Study the drawing (mm; zero at the part's minimum x, y, z) and answer. A direction names the side the tool comes from. Give positions to 0.01 mm unless a question says otherwise; leave off trailing zeros. Write each loop counter-clockwise with the first axis right and the second up, starting at its lowest first coordinate (ties: lowest second). Pieces come first, ordered by that corner, then holes. Notation, with made-up numbers: M -17,-40 L 28,-40 A15 ccw 28,-14 Z; hole C 73,-0.5 d11. An arc over 180 degrees is marked long. Use a Markdown table: item, result. Add a question column.
Item 1: A cutting plane is placed at C-C on z = 18.5. Determine the outline of the cut face in (x, y), then the cut area to 3 significant figures.
Item 2: A cutting plane is placed at B-B on x = 32. Determine the outline of the cut face in (y, z), then the cut area to 3 significant figures.
Item 3: Given P1, Ø14, axis at x = 33.5, y = 7.5, coming from the +Z side; P2, Ø12, axis at x = 24, y = 6.5, coming from the +Z side, each flat-ended and moving along its own axis, determine where each tip first touches the part or whether it passes through.
Item 4: Consider probe 1 along Z at (x, y) = (32, 20.25); probe 2 along X at (y, z) = (20.5, 21) (1 decimal); probe 3 along X at (y, z) = (3.75, 23) (1 decimal). Determine where each line is inside the solid, lowest interval first. Write a range as [from, to].
Item 5: For the marked faces 4 and 5, determine the directions among +Z, -Z, +X, -X, +Y, -Y from which every point of the face is accessible in a straight line to the end or side of a thin tool.
Item 6: A cutting plane is placed at A-A on y = 6. Determine the outline of the cut face in (x, z).
Item 7: The mould has two halves that part along Y. Classify the marked faces 1, 2 and 3: pulls with the +Y half, pulls with the -Y half, needs draft (parallel to the pull), parting line crosses it, or undercut.
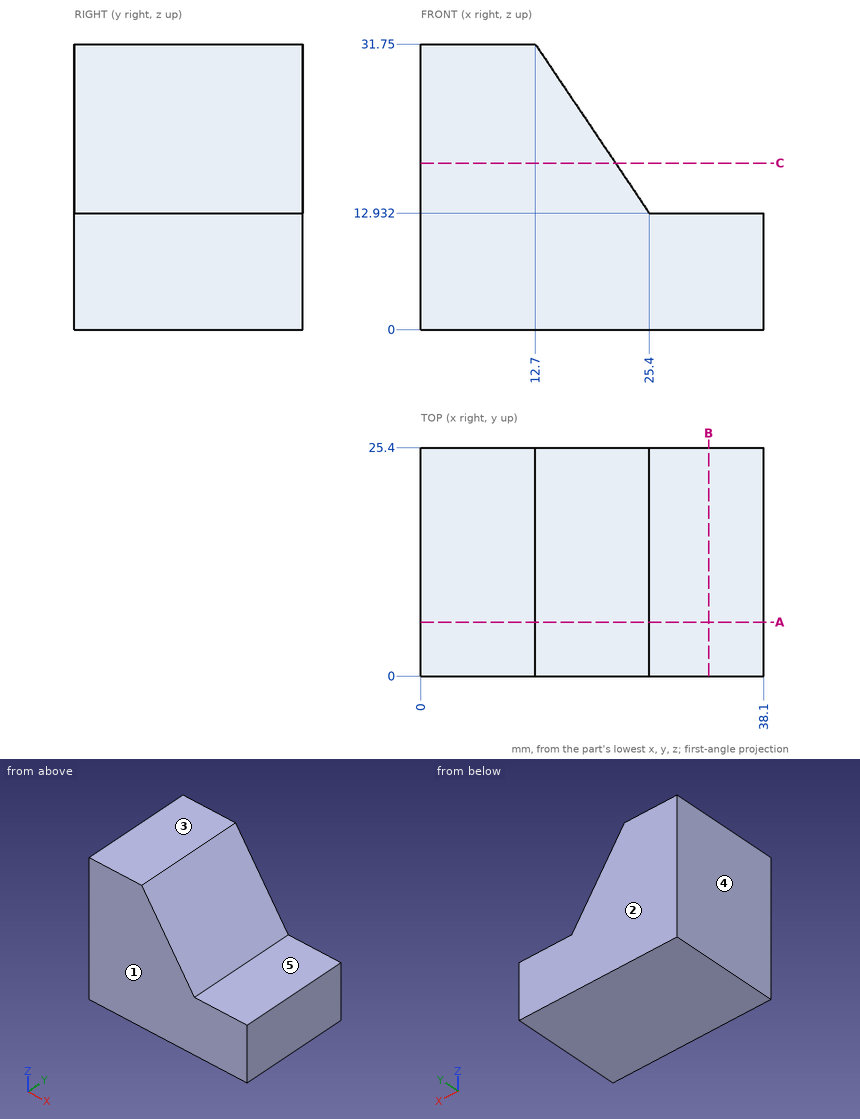
Filled in:
| question | item | result |
|---|---|---|
| 1 | outline | M 0,0 L 21.64,0 L 21.64,25.4 L 0,25.4 Z |
| 1 | area | 550 mm² |
| 2 | outline | M 0,0 L 25.4,0 L 25.4,12.93 L 0,12.93 Z |
| 2 | area | 328 mm² |
| 3 | P1 | z = 12.93 |
| 3 | P2 | z = 23.9 |
| 4 | probe 1 | [0, 12.93] |
| 4 | probe 2 | [0, 20] |
| 4 | probe 3 | [0, 18.6] |
| 5 | face 4 | +Z, -Z, -X, +Y, -Y |
| 5 | face 5 | +Z, +X, +Y, -Y |
| 6 | outline | M 0,0 L 38.1,0 L 38.1,12.93 L 25.4,12.93 L 12.7,31.75 L 0,31.75 Z |
| 7 | face 1 | pulls with the -Y half |
| 7 | face 2 | pulls with the +Y half |
| 7 | face 3 | needs draft |
